Job drawing, mm, ordinate dimensions from the low corner. One solid piece. Coordinates: 2 decimals unless noted, no trailing zeros. Loops run counter-clockwise (first coordinate to the right, second up) from the corner with the lowest first, then second, coordinate; pieces in that order, holes last. Notation, with made-up numbers: (73.25, 77.25) - (123.25, 77.25) arc R7 ccw to (123.25, 88.25) - close; hole circle Ø7 at (-20, -20). An arc over 180 degrees is marked (long way). Use a Markdown table: item, result. Add a question column.
1) Probe probe 1 along X at (y, z) = (37, 0.85); probe 2 along Y at (x, z) = (17.5, 3.95); probe 3 along X at (y, z) = (17.5, 3.3). List the from-to ranges inside material, lowest first. Write a range as [from, to].
2) Pull direction X, two halves, no side cores. Call the marked faces 1 and 2: +X half, -X half, draft (parallel to the pull), parting line (faces both ways), or undercut.
3) Band-saw the part on D-D (y = 13). Give the cut face in (x, z), plus the area to 3 significant figures.
4) Band-saw the part on B-B (z = 1.4). Give the number of separate pieces and of enclosed holes in the cut face, plus the area to 3 significant figures.
5) Drop a flat-ended pin along its axis: P1, Ø11, axis at x = 32, y = 17.5, coming from the +Z side. Give the stop position or say it passes through.
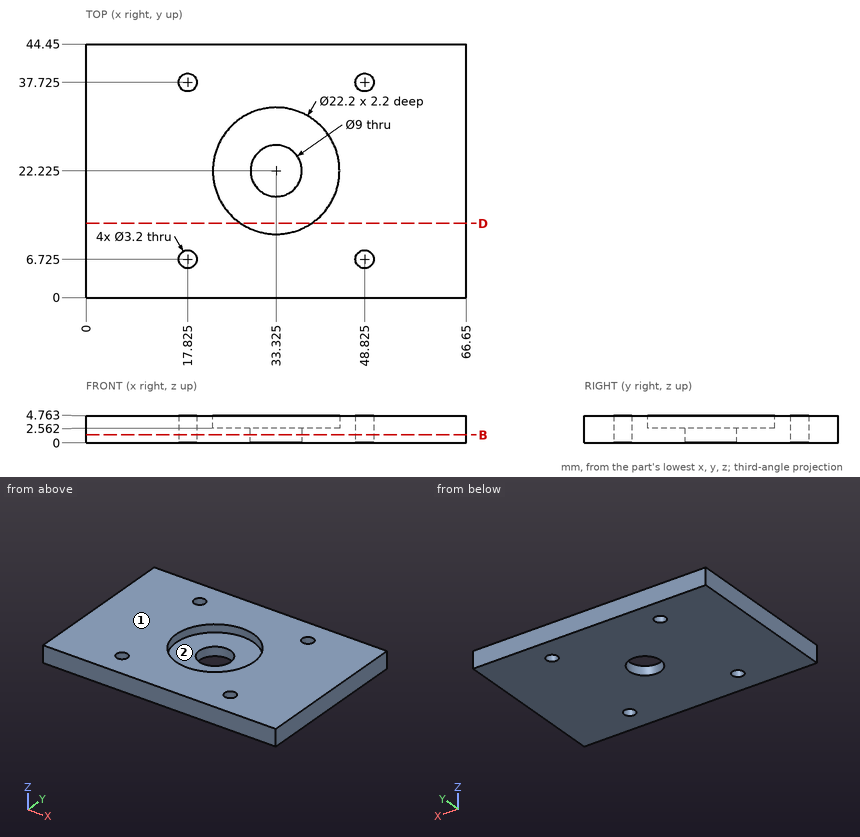
Answer block:
| question | item | result |
|---|---|---|
| 1 | probe 1 | [0, 16.4], [19.25, 47.4], [50.25, 66.65] |
| 1 | probe 2 | [0, 5.16], [8.29, 36.16], [39.29, 44.45] |
| 1 | probe 3 | [0, 23.28], [43.37, 66.65] |
| 2 | face 1 | draft |
| 2 | face 2 | undercut |
| 3 | outline | (0, 0) - (66.65, 0) - (66.65, 4.76) - (39.5, 4.76) - (39.5, 2.56) - (27.15, 2.56) - (27.15, 4.76) - (0, 4.76) - close |
| 3 | area | 290 mm2 |
| 4 | separate pieces | 1 |
| 4 | enclosed holes | 5 |
| 4 | area | 2,870 mm2 |
| 5 | P1 | z = 2.56 |
